Geometry check sheet. Reference: the model listing, model coordinates, mm. A direction names the side the tool comes from. Round coordinates to 2 decimals unless told otherwise and drop trailing zeros. Order: outer loops, then holes, each group sorted by start corner. A loop starts at its lowest first (then second) coordinate and runs counter-clockwise, first axis right, second up. Notation, with made-up numbers: (16.5, -30) - (53.5, -30) arc R27 ccw to (53.5, 0) - close; hole circle Ø5 at (25, 46.25). An arc over 180 degrees is marked (long way). Write each question's results on one line, items separated by ' | '.
```python
from build123d import *

# Parameters (mm, degrees)
SKETCH2_W             = 25.5
SKETCH2_H             = 12
BOSS_EXTRUDE1_DEPTH   = 2
SKETCH3_W             = 6.45
SKETCH3_H             = 6.45
BOSS_EXTRUDE2_DEPTH   = 2
M3X0_5_TAPPED_HOLE1_D = 2.5


with BuildPart() as part:
    # Sketch2 → Boss-Extrude1 (new body)
    with BuildSketch(Plane(origin=(0, 0, 0), x_dir=(1, 0, 0), z_dir=(0, 1, 0))):
        Rectangle(SKETCH2_W, SKETCH2_H)
    extrude(amount=BOSS_EXTRUDE1_DEPTH)

    # Sketch3 → Boss-Extrude2 (add)
    with BuildSketch(Plane(origin=(0, 2, 0), x_dir=(1, 0, 0), z_dir=(0, 1, 0))):
        with Locations((-9.525, 0)):
            Rectangle(SKETCH3_W, SKETCH3_H)
        with Locations((9.525, 0)):
            Rectangle(SKETCH3_W, SKETCH3_H)
    extrude(amount=BOSS_EXTRUDE2_DEPTH)

    # M3x0.5 Tapped Hole1 (through all)
    with Locations(Plane(origin=(0, 4, 0), x_dir=(1, 0, 0), z_dir=(0, 1, 0))):
        with Locations((-9.525, 0), (9.525, 0)):
            Hole(M3X0_5_TAPPED_HOLE1_D / 2)


solid = part.part
```
(1) Section check D-D (x = 10.5). Record the cut outline in (y, z) (3 decimals), then the cut area to 3 significant figures.
Answers follow:
outline: (0, -6) - (2, -6) - (2, -3.225) - (4, -3.225) - (4, -0.782) - (0, -0.782) - close; (0, 0.782) - (4, 0.782) - (4, 3.225) - (2, 3.225) - (2, 6) - (0, 6) - close | area: 30.6 mm²
(2) Section check B-B (y = 3.7). Record the cut outline in (x, z) (3 decimals), then the cut area to 3 significant figures.
Answers follow:
outline: (-12.75, -3.225) - (-6.3, -3.225) - (-6.3, 3.225) - (-12.75, 3.225) - close; (6.3, -3.225) - (12.75, -3.225) - (12.75, 3.225) - (6.3, 3.225) - close; hole circle Ø2.5 at (-9.525, 0); hole circle Ø2.5 at (9.525, 0) | area: 73.4 mm²
(3) Section check A-A (z = 0). Record the cut outline in (x, y) (3 decimals).
Answers follow:
outline: (-12.75, 0) - (-10.775, 0) - (-10.775, 4) - (-12.75, 4) - close; (-8.275, 0) - (8.275, 0) - (8.275, 4) - (6.3, 4) - (6.3, 2) - (-6.3, 2) - (-6.3, 4) - (-8.275, 4) - close; (10.775, 0) - (12.75, 0) - (12.75, 4) - (10.775, 4) - close
(4) Depth check by flat-ended pin: pin 1 Ø1 at (x, y) = (10, 3) entering from -Z (3 decimals); pin 2 Ø0.6 at (x, y) = (-9.5, 3.5) entering from +Z (3 decimals). Enter the tip coordinate at first touch or a pass-through.
Answers follow:
pin 1: z = -3.225 | pin 2: z = 3.225
(5) Access from +Z, -Z, +X, -X, +Y, -Y to the whole of each face (thin tool, end or side, straight path). Record for faces 4 (the face through (-10, 3, 3.225)), 5 (the face through (6.3, 3, 0)), 6 (the face through (-10, 3, -3.225)).
Answers follow:
face 4: +Z, +X, -X, +Y | face 5: +Z, -Z, +Y | face 6: -Z, +X, -X, +Y
(6) Section check C-C (z = 2). Record the cut outline in (x, y).
Answers follow:
outline: (-12.75, 0) - (12.75, 0) - (12.75, 4) - (6.3, 4) - (6.3, 2) - (-6.3, 2) - (-6.3, 4) - (-12.75, 4) - close
(7) Material ranges on line 1 (Z direction, x = -9.5, y = 3.1) (3 decimals); line 2 (X direction, y = 1.55, z = -1) (3 decimals); line 3 (X direction, y = 2.4, z = -2.5), recorded low to high.
Answers follow:
line 1: -3.225 to -1.25, 1.25 to 3.225 | line 2: -12.75 to -10.275, -8.775 to 8.775, 10.275 to 12.75 | line 3: -12.75 to -6.3, 6.3 to 12.75
(8) Draft check along X on faces 1 (the face through (-6.3, 3, 0)), 2 (the face through (12.75, 2, 0)), 3 (the face through (0, 0, 0)). Enter one of: released by +X, released by -X, zero draft, split by the parting line, or undercut.
Answers follow:
face 1: undercut | face 2: released by +X | face 3: zero draft
